Model file for the job. Use its own axes, mm. A direction names the side the tool comes from. Give positions to 0.01 mm unless a question says otherwise; leave off trailing zeros. Order: outer loops, then holes, each group sorted by start corner. A loop starts at its lowest first (then second) coordinate and runs counter-clockwise, first axis right, second up. Notation, with made-up numbers: (77, 31) - (103, 31) arc R21 cw to (103, 45) - close; hole circle Ø10 at (88.25, 33.25). An arc over 180 degrees is marked (long way). Use CSV: the item, a comma, the result in double quotes. Start each with the question number.
(1) Band-saw the part on C-C, the plane z = 5.5. Give the cut face in (x, y), then the cut area to 3 significant figures.
(2) Band-saw the part on D-D, the plane z = 19.5. Give the cut face in (x, y), then the cut area to 3 significant figures.
(3) Tool access for faces 4 (the cylindrical face through (0.867, 3.905, 37.678)), 5 (the cylindrical face through (0.867, -3.905, 0.986)), 6 (the flat face through (0, 0, 61)): list every direction of +Z, -Z, +X, -X, +Y, -Y with a clear straight run to the whole face (end or side of a thin tool).
(4) Drop flat-ended pins along their axis: pin 1 Ø9 at (x, y) = (0.5, 0.5) entering from -Z; pin 2 Ø6 at (x, z) = (2, 50.5) entering from +Y; pin 3 Ø10 at (x, z) = (3.5, 21.5) entering from -Y; pin 4 Ø5 at (x, z) = (-4, 19) entering from -Y. Give the stop position or say it passes through.
(5) Pull direction Y, two halves, no side cores. Call faces 1 (the flat face through (0, 0, 2)), 2 (the cylindrical face through (-1.08, -4.88, 11.45)), 3 (the flat face through (6, 0, 8)): +Y half, -Y half, draft (parallel to the pull), parting line (faces both ways), or undercut.
(6) Probe L1, parallel to Y at x = 0, z = 0.9; L2, parallel to Z at x = -13, y = -20; L3, parallel to Y at x = 11, z = 4.5. List the from-to ranges inside material, lowest first.
(7) Band-saw the part on A-A, the plane y = 0. Give the cut face in (x, z).
from build123d import *

# Parameters (mm, degrees)
ESQUISSE1_R             = 28.85
BOSS_EXTRU_1_DEPTH      = 8
ESQUISSE3_R             = 4
ENL_V_MAT_EXTRU_1_DEPTH = 2
ESQUISSE2_R             = 5
ESQUISSE2_R_2           = 4
BOSS_EXTRU_2_DEPTH      = 7
ESQUISSE2_2_R           = 5
ESQUISSE2_2_R_2         = 4
BOSS_EXTRU_3_DEPTH      = 2
ESQUISSE2_3_R           = 5
ESQUISSE2_3_R_2         = 4
BOSS_EXTRU_4_DEPTH      = 4
ESQUISSE4_R             = 4
BOSS_EXTRU_6_DEPTH      = 53


with BuildPart() as part:
    # Esquisse1 → Boss.-Extru.1 (new body)
    with BuildSketch(Plane.XY):
        Circle(ESQUISSE1_R)
    extrude(amount=BOSS_EXTRU_1_DEPTH)

    # Esquisse3 → Enl_v. mat.-Extru.1 (cut)
    with BuildSketch(Plane(origin=(0, 0, 0), x_dir=(-1, 0, 0), z_dir=(0, 0, -1))):
        Circle(ESQUISSE3_R)
    extrude(amount=-ENL_V_MAT_EXTRU_1_DEPTH, mode=Mode.SUBTRACT)

    # Esquisse2 → Boss.-Extru.2 (add)
    with BuildSketch(Plane.XY.offset(8)):
        Circle(ESQUISSE2_R)
        with Locations(Location((0, 0, 0), (0, 0, 180))):
            Circle(ESQUISSE2_R_2, mode=Mode.SUBTRACT)
    extrude(amount=BOSS_EXTRU_2_DEPTH)

    # Esquisse2_2 → Boss.-Extru.3 (add)
    with BuildSketch(Plane.XY.offset(8)):
        Circle(ESQUISSE2_2_R)
        with Locations(Location((0, 0, 0), (0, 0, 180))):
            Circle(ESQUISSE2_2_R_2, mode=Mode.SUBTRACT)
    extrude(amount=BOSS_EXTRU_3_DEPTH)

    # Esquisse2_3 → Boss.-Extru.4 (add)
    with BuildSketch(Plane.XY.offset(8)):
        Circle(ESQUISSE2_3_R)
        with Locations(Location((0, 0, 0), (0, 0, 180))):
            Circle(ESQUISSE2_3_R_2, mode=Mode.SUBTRACT)
    extrude(amount=BOSS_EXTRU_4_DEPTH)

    # Esquisse4 → Boss.-Extru.6 (add)
    with BuildSketch(Plane.XY.offset(8)):
        with Locations(Location((0, 0, 0), (0, 0, 180))):
            Circle(ESQUISSE4_R)
    extrude(amount=BOSS_EXTRU_6_DEPTH)


solid = part.part
Answer block:
1,outline,"circle Ø57.7 at (0, 0)"
1,area,"2,610 mm2"
2,outline,"circle Ø8 at (0, 0)"
2,area,"50.3 mm2"
3,face 4,"+Z"
3,face 5,"-Z"
3,face 6,"+Z, +X, -X, +Y, -Y"
4,pin 1,"stops at z = 0"
4,pin 2,"stops at y = 4"
4,pin 3,"stops at y = -4"
4,pin 4,"stops at y = -3.71"
5,face 1,"undercut"
5,face 2,"parting line"
5,face 3,"draft"
6,L1,"y = -28.85 to -4, 4 to 28.85"
6,L2,"z = 0 to 8"
6,L3,"y = -26.67 to 26.67"
7,outline,"(-28.85, 0) - (-4, 0) - (-4, 2) - (4, 2) - (4, 0) - (28.85, 0) - (28.85, 8) - (5, 8) - (5, 15) - (4, 15) - (4, 61) - (-4, 61) - (-4, 15) - (-5, 15) - (-5, 8) - (-28.85, 8) - close"
